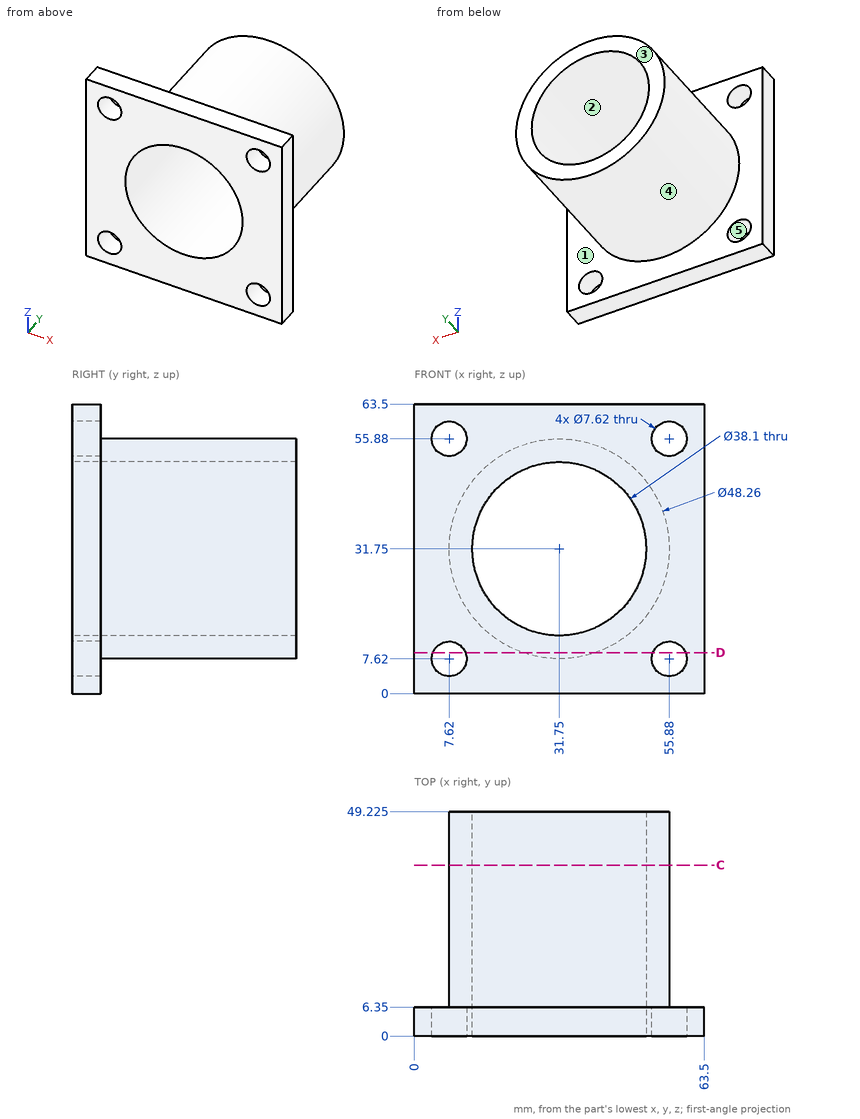
Source: three-view drawing plus pictorial views. Frame: mm from the lowest corner of the part. A direction names the side the tool comes from. Give positions to 0.01 mm unless a question says otherwise; leave off trailing zeros. Write each loop counter-clockwise with the first axis right and the second up, starting at its lowest first coordinate (ties: lowest second). Pieces come first, ordered by that corner, then holes.
(1) Cut plane C-C, the plane y = 37.5. Return loops of the section in (x, z), then the cut area to 3 significant figures.
(2) Access query for the marked faces 1 and 2. Directions: +Z, -Z, +X, -X, +Y, -Y. A direction counts if a zero-diameter tool reaches every point of the face in a straight line with its end or side. Return the directions, or none.
(3) Mould query, pull axis X, two halves, no side actions, for the marked faces 3, 4 and 5. Classes: released by +X, released by -X, zero draft, split by the parting line, or undercut.
(4) Cut plane D-D, the plane z = 9. Give the number of separate pieces and of enclosed holes in the cut face, then the cut area to 3 significant figures.
(5) Ray query, line 1 (Z direction, x = 7.62, y = 4); line 2 (X direction, y = 32.5, z = 32.5) (1 decimal); line 3 (X direction, y = 4, z = 7). Return the intervals inside material, ascending.
(6) First-contact query: P1, Ø12, axis at x = 37, y = 16, coming from the -Z side; P2, Ø1, axis at x = 30, y = 31.5, coming from the +Z side; P3, Ø4, axis at y = 33.5, z = 8.5, coming from the -X side. Flat tips, straight axial feed; report the tip coordinate or a pass-through.
Values follow:
1. outline: circle Ø48.26 at (31.75, 31.75); hole circle Ø38.1 at (31.75, 31.75)
1. area: 689 mm2
2. face 1: +Y
2. face 2: +Y, -Y
3. face 3: zero draft
3. face 4: split by the parting line
3. face 5: undercut
4. separate pieces: 3
4. enclosed holes: 0
4. area: 1,000 mm2
5. line 1: z = 0 to 3.81, 11.43 to 52.07, 59.69 to 63.5
5. line 2: x = 7.6 to 12.7, 50.8 to 55.9
5. line 3: x = 0 to 3.86, 11.38 to 52.12, 59.64 to 63.5
6. P1: stops at z = 7.62
6. P2: stops at z = 55.85
6. P3: stops at x = 20.32
